```python
from build123d import *

# Parameters (mm, degrees)
SKETCH_W        = 20
SKETCH_H        = 10
SKETCH_R        = 2.35
PAD_DEPTH       = 10
POCKET_DEPTH    = 10
POCKET001_DEPTH = 10
FILLET_R        = 1
FILLET001_R     = 1


with BuildPart() as part:
    # Sketch → Pad (new body)
    with BuildSketch(Plane.XY):
        Rectangle(SKETCH_W, SKETCH_H)
        with Locations((-5, 0)):
            Circle(SKETCH_R, mode=Mode.SUBTRACT)
        with Locations((5, 0)):
            Circle(SKETCH_R, mode=Mode.SUBTRACT)
    extrude(amount=PAD_DEPTH)

    # Sketch001 → Pocket (cut)
    with BuildSketch(Plane.XY):
        Polygon((-5, 0), (-6.5, -5), (-3.5, -5), align=None)
    extrude(amount=POCKET_DEPTH, mode=Mode.SUBTRACT)

    # MirroredSketch → Pocket001 (cut)
    with BuildSketch(Plane.XY):
        Polygon((5, 0), (6.5, -5), (3.5, -5), align=None)
    extrude(amount=POCKET001_DEPTH, mode=Mode.SUBTRACT)

    # Fillet
    fillet_edges = [part.edges().sort_by_distance(p)[0] for p in [
        (-6.5, -5, 5),
    ]]
    fillet(fillet_edges, radius=FILLET_R)

    # Fillet001
    fillet001_edges = [part.edges().sort_by_distance(p)[0] for p in [
        (-10, -5, 5),
        (-3.5, -5, 5),
        (3.5, -5, 5),
        (6.5, -5, 5),
        (10, -5, 5),
        (10, 5, 5),
        (-10, 5, 5),
    ]]
    fillet(fillet001_edges, radius=FILLET001_R)


solid = part.part
```
Can you work these out from the model? Positions are in its coordinate system, mm. A direction names the side the tool comes from. Round coordinates to 2 decimals unless told otherwise and drop trailing zeros. Order: outer loops, then holes, each group sorted by start corner. A loop starts at its lowest first (then second) coordinate and runs counter-clockwise, first axis right, second up.
(1) On a 3-axis mill with a long thin cutter (end or side, diameter ignored), from which of +Z, -Z, +X, -X, +Y, -Y can I reach the whole of each face in a straight line? I mean faces 1 (the face through (-5.976, -3.255, 4.93)), 2 (the face through (-8, -5, 5)). Say none if no direction works.
Results are:
face 1: +Z, -Z, -Y
face 2: +Z, -Z, +X, -X, -Y
(2) I'm going to push a flat-ended pin straight in: pin 1 (4 mm diameter, centred on x = 5, y = 0, fed in from +Z). Where does the tip first touch, or does it pass through?
Results are:
pin 1: passes through
(3) If we section it at B-B (y = 0): Please give me the cut outline in (x, z).
Results are:
outline: (-10, 0) - (-7.35, 0) - (-7.35, 10) - (-10, 10) - close; (-2.65, 0) - (2.65, 0) - (2.65, 10) - (-2.65, 10) - close; (7.35, 0) - (10, 0) - (10, 10) - (7.35, 10) - close
(4) If we section it at D-D (x = -5): Please give me the cut outline in (y, z).
Results are:
outline: (2.35, 0) - (5, 0) - (5, 10) - (2.35, 10) - close
(5) If we section it at A-A (z = 3.75): Please give me the cut outline in (x, y).
Results are:
outline: (-10, -4) arc R1 ccw to (-9, -5) - (-7.24, -5) arc R1 ccw to (-6.29, -4.29) - (-5.68, -2.25) arc R2.35 cw (long way) to (-4.32, -2.25) - (-3.71, -4.29) arc R1 ccw to (-2.76, -5) - (2.76, -5) arc R1 ccw to (3.71, -4.29) - (4.32, -2.25) arc R2.35 cw (long way) to (5.68, -2.25) - (6.29, -4.29) arc R1 ccw to (7.24, -5) - (9, -5) arc R1 ccw to (10, -4) - (10, 4) arc R1 ccw to (9, 5) - (-9, 5) arc R1 ccw to (-10, 4) - close
(6) If we section it at C-C (x = 7): Please give me the cut outline in (y, z), plus the area to 3 significant figures.
Results are:
outline: (-4.97, 0) - (-1.23, 0) - (-1.23, 10) - (-4.97, 10) - close; (1.23, 0) - (5, 0) - (5, 10) - (1.23, 10) - close
area: 75.0 mm2
(7) We'd pull the mould along X, two halves only. Please class faces 3 (the face through (-6.64, -4.797, 5.07)), 4 (the face through (0, -5, 5)), 5 (the face through (-9.715, 4.699, 5.07)), 6 (the face through (9.699, 4.715, 5.07)): +X half, -X half, draft (parallel to the pull), parting line (faces both ways), or undercut.
Results are:
face 3: undercut
face 4: draft
face 5: -X half
face 6: +X half
(8) If I drill on L1, parallel to X at y = 0, z = 3; L2, parallel to X at y = -1.75, z = 0.5; L3, parallel to Y at x = 5, z = 5, over which ranges is the centre line in solid material (lowest first)?
Results are:
L1: x = -10 to -7.35, -2.65 to 2.65, 7.35 to 10
L2: x = -10 to -6.57, -3.43 to 3.43, 6.57 to 10
L3: y = 2.35 to 5
